Read the model definition and answer for the solid it produces. Units are mm, in the model's axes. A direction names the side the tool comes from. Coordinates: 2 decimals unless noted, no trailing zeros. Order: outer loops, then holes, each group sorted by start corner. A loop starts at its lowest first (then second) coordinate and runs counter-clockwise, first axis right, second up. Notation, with made-up numbers: (-20, -5) -> (20, -5) arc R20 ccw to (20, 4) -> close; hole circle Ø11 at (-23, -28). An arc over 180 degrees is marked (long way). Return JSON: item names as keys, results as strings. Group by question number.
```python
from build123d import *

# Parameters (mm, degrees)
SKETCH2_W                                       = 10
SKETCH2_H                                       = 44
BOSS_EXTRUDE3_DEPTH                             = 2.5
F_2_0MM_DOWEL_SLOT3_D                           = 2
SKETCH18_W                                      = 10
SKETCH18_H                                      = 2.5
BOSS_EXTRUDE4_DEPTH                             = 2.5
SKETCH19_W                                      = 10
SKETCH19_H                                      = 2.5
BOSS_EXTRUDE5_DEPTH                             = 2.5
SKETCH20_W                                      = 10
SKETCH20_H                                      = 2.5
BOSS_EXTRUDE6_DEPTH                             = 14.5
SKETCH22_W                                      = 10
SKETCH22_H                                      = 2.5
BOSS_EXTRUDE7_DEPTH                             = 10
SKETCH23_W                                      = 10
SKETCH23_H                                      = 2.5
BOSS_EXTRUDE8_DEPTH                             = 10
CSK_FOR_M2_FLAT_HEAD_MACHINE_SCREW1_D           = 2.4
CSK_FOR_M2_FLAT_HEAD_MACHINE_SCREW1_CSINK_D     = 4.4
CSK_FOR_M2_FLAT_HEAD_MACHINE_SCREW1_CSINK_ANGLE = 90
CSK_FOR_M2_FLAT_HEAD_MACHINE_SCREW2_D           = 2.4
CSK_FOR_M2_FLAT_HEAD_MACHINE_SCREW2_CSINK_D     = 4.4
CSK_FOR_M2_FLAT_HEAD_MACHINE_SCREW2_CSINK_ANGLE = 90


with BuildPart() as part:
    # Sketch2 → Boss-Extrude3 (new body)
    with BuildSketch(Plane(origin=(0, 0, 0), x_dir=(1, 0, 0), z_dir=(0, 1, 0))):
        with Locations((-1.558139535, -13.697674419)):
            Rectangle(SKETCH2_W, SKETCH2_H)
    extrude(amount=BOSS_EXTRUDE3_DEPTH)

    # Ø2.0mm Dowel Slot3 (through all)
    with Locations(Plane(origin=(0, 2.5, 0), x_dir=(1, 0, 0), z_dir=(0, 1, 0))):
        with Locations((-4.058139535, 4.302325581), (-4.058139535, 0.302325581), (-4.058139535, -3.697674419), (-4.058139535, -7.697674419), (-4.058139535, -11.697674419), (-4.058139535, -15.697674419), (-4.058139535, -19.697674419), (-4.058139535, -23.697674419), (-4.058139535, -27.697674419), (-4.058139535, -31.697674419), (0.941860465, 2.302325581), (0.941860465, -1.697674419), (0.941860465, -5.697674419), (0.941860465, -9.697674419), (0.941860465, -13.697674419), (0.941860465, -17.697674419), (0.941860465, -21.697674419), (0.941860465, -25.697674419), (0.941860465, -29.697674419), (0.941860465, -33.697674419), (0.941860465, 6.302325581)):
            Hole(F_2_0MM_DOWEL_SLOT3_D / 2)

    # Sketch18 → Boss-Extrude4 (add)
    with BuildSketch(Plane.XY.offset(35.697674419)):
        with Locations((-1.558139535, 1.25)):
            Rectangle(SKETCH18_W, SKETCH18_H)
    extrude(amount=BOSS_EXTRUDE4_DEPTH)

    # Sketch19 → Boss-Extrude5 (add)
    with BuildSketch(Plane(origin=(0, 0, -8.302325581), x_dir=(-1, 0, 0), z_dir=(0, 0, -1))):
        with Locations((1.558139535, 1.25)):
            Rectangle(SKETCH19_W, SKETCH19_H)
    extrude(amount=BOSS_EXTRUDE5_DEPTH)

    # Sketch20 → Boss-Extrude6 (add)
    with BuildSketch(Plane.XZ):
        with Locations((-1.558139535, 36.947674419)):
            Rectangle(SKETCH20_W, SKETCH20_H)
        with Locations((-1.558139535, -9.552325581)):
            Rectangle(SKETCH20_W, SKETCH20_H)
    extrude(amount=BOSS_EXTRUDE6_DEPTH)

    # Sketch22 → Boss-Extrude7 (add)
    with BuildSketch(Plane(origin=(0, 0, -10.802325581), x_dir=(-1, 0, 0), z_dir=(0, 0, -1))):
        with Locations((1.558139535, -13.25)):
            Rectangle(SKETCH22_W, SKETCH22_H)
    extrude(amount=BOSS_EXTRUDE7_DEPTH)

    # Sketch23 → Boss-Extrude8 (add)
    with BuildSketch(Plane.XY.offset(38.197674419)):
        with Locations((-1.558139535, -13.25)):
            Rectangle(SKETCH23_W, SKETCH23_H)
    extrude(amount=BOSS_EXTRUDE8_DEPTH)

    # CSK for M2 Flat Head Machine Screw1 (through all)
    with Locations(Plane(origin=(0, -12, 0), x_dir=(1, 0, 0), z_dir=(0, 1, 0))):
        with Locations((-1.558139535, 15.802325581)):
            CounterSinkHole(CSK_FOR_M2_FLAT_HEAD_MACHINE_SCREW1_D / 2, CSK_FOR_M2_FLAT_HEAD_MACHINE_SCREW1_CSINK_D / 2, counter_sink_angle=CSK_FOR_M2_FLAT_HEAD_MACHINE_SCREW1_CSINK_ANGLE)

    # CSK for M2 Flat Head Machine Screw2 (through all)
    with Locations(Plane(origin=(0, -12, 0), x_dir=(1, 0, 0), z_dir=(0, 1, 0))):
        with Locations((-1.558139535, -43.197674419)):
            CounterSinkHole(CSK_FOR_M2_FLAT_HEAD_MACHINE_SCREW2_D / 2, CSK_FOR_M2_FLAT_HEAD_MACHINE_SCREW2_CSINK_D / 2, counter_sink_angle=CSK_FOR_M2_FLAT_HEAD_MACHINE_SCREW2_CSINK_ANGLE)


solid = part.part
```
1. For a pull along X with two mould halves and no side action, classify faces 4 (the face through (-0.67, -13.76, 42.39)), 5 (the face through (1, -12, -16)), 6 (the face through (-6.558, 0.3, 13.5)) as released by +X, released by -X, zero draft, split by the parting line, or undercut.
2. Find section A-A on y = -10.75. Determine the outline of the cut face in (x, z).
3. Given pin 1 (1.8 mm diameter, centred on x = 0.94, z = -2.3, fed in from +Y); pin 2 (5 mm diameter, centred on x = 0, y = -3, fed in from -Z); pin 3 (2.5 mm diameter, centred on x = 0.94, z = 25.7, fed in from -Y), each flat-ended and moving along its own axis, determine where each tip first touches the part or whether it passes through.
4. Straight lines are drawn through the part: L1, parallel to Z at x = -5.5, y = -7.25; L2, parallel to Z at x = -2.5, y = -12.25; L3, parallel to Y at x = -6, z = 1. For each, find the intervals that lie inside material, in ascending order.
5. Find section B-B on y = 0.75. Give the number of separate pieces and of enclosed holes in the cut face, and give its area (3 significant figures).
6. Which of the six approach directions +Z, -Z, +X, -X, +Y, -Y give full straight-line access (tool end or side, diameter ignored) to faces 1 (the face through (-3.928, 1.233, 26.706)), 2 (the face through (-4, -12, 43)), 3 (the face through (-1, -5, -10.802))?
Result:
{
 "1": {"face 4": "undercut", "face 5": "zero draft", "face 6": "released by -X"},
 "2": {"outline": "(-6.56, -10.8) -> (3.44, -10.8) -> (3.44, -8.3) -> (-6.56, -8.3) -> close; (-6.56, 35.7) -> (3.44, 35.7) -> (3.44, 38.2) -> (-6.56, 38.2) -> close"},
 "3": {"pin 1": "through", "pin 2": "z = -10.8", "pin 3": "y = 0"},
 "4": {"L1": "-10.8 to -8.3, 35.7 to 38.2", "L2": "-20.8 to -17.51, -14.09 to -8.3, 35.7 to 41.49, 44.91 to 48.2", "L3": "0 to 2.5"},
 "5": {"separate pieces": "1", "enclosed holes": "21", "area": "424 mm^2"},
 "6": {"face 1": "+Y, -Y", "face 2": "+Z, +X, -X, +Y", "face 3": "-Z, +X, -X, +Y"}
}
